```python
from build123d import *

# Parameters (mm, degrees)
F1_DEPTH = 63.5
F2_DEPTH = 25.4
F3_DEPTH = 7.9375
F0_W     = 25.4
F0_H     = 19.05
F4_DEPTH = 25.4
F6_R     = 6.35


# Not quite as in the source:
# - a feature names something its author has since deleted; it is built from what else it names


with BuildPart() as f1:
    # F0 (on Front) → F1 (new body, symmetric)
    with BuildSketch(Plane.XZ):
        Polygon((22.225, 9.525), (-41.275, 9.525), (-41.275, -9.525), (41.275, -9.525), (41.275, 9.525), align=None)
    extrude(amount=F1_DEPTH, both=True)

    # F0 (on Front) → F2 (join, symmetric)
    with BuildSketch(Plane.XZ):
        with BuildLine():
            Line((22.225, 27.0002), (22.225, 9.525))
            Line((22.225, 9.525), (41.275, 9.525))
            Line((41.275, 9.525), (41.275, 27.0002))
            ThreePointArc((41.275, 27.0002), (45.9246798487, 38.2255201513), (57.15, 42.8752))
            Line((57.15, 42.8752), (60.325, 42.8752))
            Line((60.325, 42.8752), (60.325, 61.9252))
            Line((60.325, 61.9252), (57.15, 61.9252))
            ThreePointArc((57.15, 61.9252), (32.4542956671, 51.6959043329), (22.225, 27.0002))
        make_face()
    extrude(amount=F2_DEPTH, both=True)

    # F0 (on Front) → F3 (join, symmetric)
    with BuildSketch(Plane.XZ):
        with BuildLine():
            add(Edge.make_bspline(
                [(-41.275, 9.525), (-28.3377878368, 47.713726759), (0, 62.2769519687), (57.15, 61.9252)],
                knots=[0, 0, 0, 0, 111.5045361635, 111.5045361635, 111.5045361635, 111.5045361635], degree=3))
            Line((-41.275, 9.525), (22.225, 9.525))
            Line((22.225, 9.525), (22.225, 27.0002))
            ThreePointArc((22.225, 27.0002), (32.4542956671, 51.6959043329), (57.15, 61.9252))
        make_face()
    extrude(amount=F3_DEPTH, both=True)

    # F0 (on Front) → F4 (join, symmetric)
    with BuildSketch(Plane.XZ):
        with Locations((73.025, 52.4002)):
            Rectangle(F0_W, F0_H)
    extrude(amount=F4_DEPTH, both=True)

    # F0 (on Front) → F5 (revolve)
    with BuildSketch(Plane.XZ):
        Polygon((85.725, 66.675), (85.725, 61.9252), (85.725, 42.8752), (85.725, 38.1), (111.125, 38.1), (111.125, 66.675), align=None)
    revolve(axis=Axis((85.725, 0, 52.3875), (0, 0, -1)))

    # F6
    f6_edges = [f1.edges().sort_by_distance(p)[0] for p in [
        (-41.275, -63.5, 0),
        (41.275, -63.5, 0),
        (41.275, 63.5, 0),
        (-41.275, 63.5, 0),
    ]]
    fillet(f6_edges, radius=F6_R)


solid = f1.part
```
The listing builds one solid part. Answer for the finished solid, in the listing's coordinates (mm). A direction names the side the tool comes from. Give positions to 0.01 mm unless a question says otherwise; leave off trailing zeros. Loops run counter-clockwise (first coordinate to the right, second up) from the corner with the lowest first, then second, coordinate; pieces in that order, holes last. Notation, with made-up numbers: (67, -36.75) - (72, -36.75) arc R27 cw to (72, -2.75) - close; hole circle Ø4 at (14.5, 44). An arc over 180 degrees is marked (long way). Answer as CSV lines item,"result". Start each with the question number.
Item 1: A cutting plane is placed at C-C on y = -44. Determine the outline of the cut face in (x, z) (3 decimals).
Item 2: Find the intervals of material crossed by line 1 (Y direction, x = 0, z = 33); line 2 (X direction, y = -53.5, z = 6) (3 decimals); line 3 (Z direction, x = 77.5, y = 19.5) (3 decimals), in increasing order. Write a range as from..to.
Item 3: A cutting plane is placed at A-A on z = -1. Determine the outline of the cut face in (x, y) (3 decimals).
Item 4: For faces 1 (the face through (32.73, 16.55, 51.97)), 2 (the face through (86, 0, 38.1)), 3 (the face through (46, 25.4, 42)), determine the directions among +Z, -Z, +X, -X, +Y, -Y from which every point of the face is accessible in a straight line to the end or side of a thin tool.
Item 5: A cutting plane is placed at B-B on y = -21. Determine the outline of the cut face in (x, z) (3 decimals), then the cut area to 3 significant figures.
Item 6: Each of these flat-tipped pins is pushed along its axis until it touches: pin 1 (6 mm diameter, centred on x = 37, z = 57, fed in from +Y); pin 2 (23 mm diameter, centred on x = 68.5, y = -5.5, fed in from -Z); pin 3 (1.5 mm diameter, centred on y = 4, z = 19.5, fed in from +X) (3 decimals). Where does it stop, or does it pass through?
Found:
1,outline,"(-41.275, -9.525) - (41.275, -9.525) - (41.275, 9.525) - (-41.275, 9.525) - close"
2,line 1,"y = -7.94..7.94"
2,line 2,"x = -41.275..41.275"
2,line 3,"z = 38.1..66.675"
3,outline,"(-41.275, -57.15) arc R6.35 ccw to (-34.925, -63.5) - (34.925, -63.5) arc R6.35 ccw to (41.275, -57.15) - (41.275, 57.15) arc R6.35 ccw to (34.925, 63.5) - (-34.925, 63.5) arc R6.35 ccw to (-41.275, 57.15) - close"
4,face 1,"+Z, -X, +Y"
4,face 2,"-Z, +X, +Y, -Y"
4,face 3,"+Z, +X, -X, +Y"
5,outline,"(-41.275, -9.525) - (41.275, -9.525) - (41.275, 27) arc R15.875 cw to (57.15, 42.875) - (71.437, 42.875) - (71.437, 38.1) - (100.013, 38.1) - (100.013, 66.675) - (71.437, 66.675) - (71.437, 61.925) - (57.15, 61.925) arc R34.925 ccw to (22.225, 27) - (22.225, 9.525) - (-41.275, 9.525) - close"
5,area,"3,750 mm^2"
6,pin 1,"stops at y = 25.4"
6,pin 2,"stops at z = 38.1"
6,pin 3,"stops at x = 41.275"
